Read the model definition and answer for the solid it produces. Units are mm, in the model's axes. A direction names the side the tool comes from. Coordinates: 2 decimals unless noted, no trailing zeros. Order: outer loops, then holes, each group sorted by start corner. A loop starts at its lowest first (then second) coordinate and runs counter-clockwise, first axis right, second up.
```python
from build123d import *

# Parameters (mm, degrees)
F1_DEPTH  = 38
F3_DEPTH  = 25
F4_DEPTH  = 38
F0_W      = 25
F0_H      = 10
F5_DEPTH  = 5
F6_DEPTH  = 10
F7_DEPTH  = 15
F0_W_2    = 5
F0_H_2    = 27
F8_DEPTH  = 38
F9_DEPTH  = 33
F10_DEPTH = 15
F11_DEPTH = 20
F0_W_3    = 10
F0_H_3    = 22
F12_DEPTH = 25
F13_DEPTH = 30


with BuildPart() as f1:
    # F0 (on Top) → F1 (new body)
    with BuildSketch(Plane.XY):
        Polygon((-45, 18.8800000995), (-50, 18.8800000995), (-50, -23.1199999005), (-45, -23.1199999005), (-45, -13.1199999005), (-45, -3.1199999005), align=None)
    extrude(amount=F1_DEPTH)

    # F2 (on face) → F3 (cut)
    with BuildSketch(Plane.YZ.offset(-45)):
        Polygon((-23.1199999005, 14), (18.8800000995, 38), (-23.1199999005, 38), align=None)
    extrude(amount=-F3_DEPTH, mode=Mode.SUBTRACT)

    # F0 (on Top) → F4 (join)
    with BuildSketch(Plane.XY):
        Polygon((0, 23.8800000995), (-50, 23.8800000995), (-50, 18.8800000995), (-45, 18.8800000995), (-20, 18.8800000995), (-10, 18.8800000995), (0, 18.8800000995), align=None)
    extrude(amount=F4_DEPTH)

    # F0 (on Top) → F5 (join)
    with BuildSketch(Plane.XY):
        with Locations((-32.5, -18.1199999005)):
            Rectangle(F0_W, F0_H)
    extrude(amount=F5_DEPTH)

    # F0 (on Top) → F6 (join)
    with BuildSketch(Plane.XY):
        Polygon((22, -13.1199999005), (22, -3.1199999005), (0, -3.1199999005), (-10, -3.1199999005), (-20, -3.1199999005), (-45, -3.1199999005), (-45, -13.1199999005), (-20, -13.1199999005), align=None)
    extrude(amount=F6_DEPTH)

    # F0 (on Top) → F7 (join)
    with BuildSketch(Plane.XY):
        Polygon((27, -3.1199999005), (22, -3.1199999005), (22, -13.1199999005), (22, -23.1199999005), (27, -23.1199999005), align=None)
    extrude(amount=F7_DEPTH)

    # F0 (on Top) → F8 (join)
    with BuildSketch(Plane.XY):
        with Locations((24.5, 10.3800000995)):
            Rectangle(F0_W_2, F0_H_2)
    extrude(amount=F8_DEPTH)

    # F0 (on Top) → F9 (join)
    with BuildSketch(Plane.XY):
        Polygon((22, 23.8800000995), (0, 23.8800000995), (0, 18.8800000995), (0, -3.1199999005), (22, -3.1199999005), align=None)
    extrude(amount=F9_DEPTH)

    # F0 (on Top) → F10 (join)
    with BuildSketch(Plane.XY):
        Polygon((-20, -3.1199999005), (-45, 18.8800000995), (-45, -3.1199999005), align=None)
    extrude(amount=F10_DEPTH)

    # F0 (on Top) → F11 (join)
    with BuildSketch(Plane.XY):
        Polygon((-20, 18.8800000995), (-45, 18.8800000995), (-20, -3.1199999005), align=None)
    extrude(amount=F11_DEPTH)

    # F0 (on Top) → F12 (join)
    with BuildSketch(Plane.XY):
        with Locations((-15, 7.8800000995)):
            Rectangle(F0_W_3, F0_H_3)
    extrude(amount=F12_DEPTH)

    # F0 (on Top) → F13 (join)
    with BuildSketch(Plane.XY):
        with Locations((-5, 7.8800000995)):
            Rectangle(F0_W_3, F0_H_3)
    extrude(amount=F13_DEPTH)


solid = f1.part
```
1) Flat-ended cylindrical pins translate along their axes: pin 1 Ø5 at (x, z) = (0, 29) entering from -Y; pin 2 Ø11 at (x, y) = (-20.5, -8) entering from +Z; pin 3 Ø4 at (x, y) = (24.5, -14.5) entering from +Z. Find the tip coordinate at first contact, or state that the pin passes through.
A:
pin 1: stops at y = -3.12
pin 2: stops at z = 25
pin 3: stops at z = 15
2) Straight lines are drawn through the part: line 1 (X direction, y = -9, z = 11.5); line 2 (X direction, y = 21, z = 34); line 3 (Z direction, x = 24, y = -12). For each, find the intervals that lie inside material, in ascending order.
A:
line 1: x = -50 to -45, 22 to 27
line 2: x = -50 to 0, 22 to 27
line 3: z = 0 to 15
3) Determine the mould class of faces 4 (the flat face through (24, -23.12, 7)), 5 (the flat face through (0, 8, 31)) for opening direction X: pulls with the +X half, pulls with the -X half, needs draft (parallel to the pull), parting line crosses it, or undercut.
A:
face 4: needs draft
face 5: undercut
4) Which of the six approach directions +Z, -Z, +X, -X, +Y, -Y give full straight-line access (tool end or side, diameter ignored) to faces 1 (the flat face through (22, 10, 35)), 2 (the flat face through (-20, -18, 2)), 3 (the flat face through (-15, 8, 25))?
A:
face 1: +Z, +Y, -Y
face 2: +Z, -Z, -Y
face 3: +Z, -Y
5) A cutting plane is placed at C-C, the plane y = 16.5. Determine the outline of the cut face in (x, z).
A:
outline: (-50, 0) - (27, 0) - (27, 38) - (22, 38) - (22, 33) - (0, 33) - (0, 30) - (-10, 30) - (-10, 25) - (-20, 25) - (-20, 20) - (-42.3, 20) - (-42.3, 15) - (-45, 15) - (-45, 36.64) - (-50, 36.64) - close
6) A cutting plane is placed at B-B, the plane x = -13. Determine the outline of the cut face in (y, z), and give its area (3 significant figures).
A:
outline: (-13.12, 0) - (23.88, 0) - (23.88, 38) - (18.88, 38) - (18.88, 25) - (-3.12, 25) - (-3.12, 10) - (-13.12, 10) - close
area: 840 mm2
7) A cutting plane is placed at D-D, the plane z = 16. Determine the outline of the cut face in (x, y), and give its area (3 significant figures).
A:
outline: (-50, -19.62) - (-45, -19.62) - (-45, 18.88) - (-20, -3.12) - (27, -3.12) - (27, 23.88) - (-50, 23.88) - close
area: 1,890 mm2
8) A cutting plane is placed at A-A, the plane z = 7.5. Determine the outline of the cut face in (x, y), and give its area (3 significant figures).
A:
outline: (-50, -23.12) - (-45, -23.12) - (-45, -13.12) - (22, -13.12) - (22, -23.12) - (27, -23.12) - (27, 23.88) - (-50, 23.88) - close
area: 2,950 mm2
